Design review of the part built by this model. Coordinates are the model's own, in mm. A direction names the side the tool comes from. Coordinates: 2 decimals unless noted, no trailing zeros. Loops run counter-clockwise (first coordinate to the right, second up) from the corner with the lowest first, then second, coordinate; pieces in that order, holes last. Notation, with made-up numbers: (70.5, -3) -> (84.5, -3) arc R16 ccw to (84.5, 27) -> close; hole circle Ø2 at (36, 27.5). An arc over 180 degrees is marked (long way). Answer as a JSON object with one key per item and string values.
```python
from build123d import *

# Parameters (mm, degrees)
F0_R     = 15.875
F0_R_2   = 1.27
F0_R_3   = 7.62
F1_DEPTH = 1.524
F0_R_4   = 1.5875
F2_DEPTH = 5.08


with BuildPart() as f1:
    # F0 (on Front) → F1 (new body)
    with BuildSketch(Plane.XZ):
        Circle(F0_R)
        with Locations((-10.173633, -5.87375)):
            Circle(F0_R_2, mode=Mode.SUBTRACT)
        with Locations((0, -11.7475)):
            Circle(F0_R_2, mode=Mode.SUBTRACT)
        with Locations((10.173633, -5.87375)):
            Circle(F0_R_2, mode=Mode.SUBTRACT)
        with Locations((-10.173633, 5.87375)):
            Circle(F0_R_2, mode=Mode.SUBTRACT)
        Circle(F0_R_3, mode=Mode.SUBTRACT)
        with Locations((10.173633, 5.87375)):
            Circle(F0_R_2, mode=Mode.SUBTRACT)
        with Locations((0, 11.7475)):
            Circle(F0_R_2, mode=Mode.SUBTRACT)
    extrude(amount=F1_DEPTH)

    # F0 (on Front) → F2 (join)
    with BuildSketch(Plane.XZ):
        Circle(F0_R_3)
        Circle(F0_R_4, mode=Mode.SUBTRACT)
    extrude(amount=F2_DEPTH)


solid = f1.part
```
1) Add section A-A, the plane x = 0. Give the boundary of the cut face in (y, z) (1 decimal).
Completed:
{"outline": "(-5.1, -7.6) -> (-1.5, -7.6) -> (-1.5, -10.5) -> (0, -10.5) -> (0, -1.6) -> (-5.1, -1.6) -> close; (-5.1, 1.6) -> (0, 1.6) -> (0, 10.5) -> (-1.5, 10.5) -> (-1.5, 7.6) -> (-5.1, 7.6) -> close; (-1.5, -15.9) -> (0, -15.9) -> (0, -13) -> (-1.5, -13) -> close; (-1.5, 13) -> (0, 13) -> (0, 15.9) -> (-1.5, 15.9) -> close"}
2) Add section C-C, the plane y = -0.7. Count the separate pieces of the cut face and the enclosed holes in it, and give its area (3 significant figures).
Completed:
{"separate pieces": "1", "enclosed holes": "7", "area": "753 mm²"}
3) Wall thickness on probe 1 along Z at (x, y) = (0, -0.85) (1 decimal); probe 2 along Z at (x, y) = (0, -3.75); probe 3 along Y at (x, z) = (-1, -10): over which ranges is each line inside the solid? List them lowest first.
Completed:
{"probe 1": "-15.9 to -13, -10.5 to -1.6, 1.6 to 10.5, 13 to 15.9", "probe 2": "-7.62 to -1.59, 1.59 to 7.62", "probe 3": "-1.52 to 0"}
4) For faces 4 (the flat face through (7, -1.524, 4)), 5 (the cylindrical face through (-9.491, -0.751, -4.803)), list the 3-axis set-ups (+Z, -Z, +X, -X, +Y, -Y) from which the entire face can be reached by the end or side of a thin tool; tool diameter is ignored.
Completed:
{"face 4": "-Y", "face 5": "+Y, -Y"}
5) Add section D-D, the plane y = -2.45. Give the boundary of the cut face in (x, z) (1 decimal).
Completed:
{"outline": "circle Ø15.2 at (0, 0); hole circle Ø3.2 at (0, 0)"}
6) The part is to be moulded in two halves that separate along Z. For faces 1 (the flat face through (2, -5.08, 0)), 2 (the cylindrical face through (10.76, -0.751, 4.747)), 3 (the cylindrical face through (-1.65, -3.28, -7.44)), say which applies: pulls with the +Z half, pulls with the -Z half, needs draft (parallel to the pull), parting line crosses it, or undercut.
Completed:
{"face 1": "needs draft", "face 2": "undercut", "face 3": "parting line crosses it"}
7) Clearance check with flat-ended pins moving along their axes: pin 1 Ø2 at (x, z) = (-10.17, 5.87) entering from +Y; pin 2 Ø3 at (x, z) = (10.17, 5.87) entering from -Y. State where each tip first meets the part, or that it passes through.
Completed:
{"pin 1": "through", "pin 2": "y = -1.52"}
8) Add section B-B, the plane z = 0. Give the boundary of the cut face in (x, y) (1 decimal), and give its area (3 significant figures).
Completed:
{"outline": "(-15.9, -1.5) -> (-7.6, -1.5) -> (-7.6, -5.1) -> (-1.6, -5.1) -> (-1.6, 0) -> (-15.9, 0) -> close; (1.6, -5.1) -> (7.6, -5.1) -> (7.6, -1.5) -> (15.9, -1.5) -> (15.9, 0) -> (1.6, 0) -> close", "area": "86.5 mm²"}
